Can you work these out from the model? Positions are in its coordinate system, mm. A direction names the side the tool comes from. Coordinates: 2 decimals unless noted, no trailing zeros. Write each loop counter-clockwise with the first axis right and the second up, starting at its lowest first coordinate (ties: lowest second). Pieces come first, ordered by that corner, then holes. Notation, with made-up numbers: (9.25, 34) - (56.25, 34) arc R29 cw to (56.25, 71) - close; hole circle Ø7 at (42.5, -37.5). An arc over 180 degrees is marked (long way). Write each question's results on one line, items separated by ' | '. Start each with the question number.
```python
from build123d import *


with BuildPart() as f1:
    # F0 (on Top) → F1 (revolve)
    with BuildSketch(Plane.XY):
        with BuildLine():
            Line((-8.1, 12.624975), (0, 0))
            Line((0, 0), (3.5, 0))
            Line((3.5, 0), (3.5, 7))
            Line((3.5, 7), (-1.81, 7))
            Line((-1.81, 7), (-1.81, 10.05))
            Line((-1.81, 10.05), (0.49, 10.05))
            Line((0.49, 10.05), (-1.356164, 21.907136))
            Line((-1.356164, 21.907136), (-12.356164, 21.907136))
            Line((-12.356164, 21.907136), (-12.356164, 21.31))
            ThreePointArc((-12.356164, 21.31), (-7.520242, 18.294486), (-8.1, 12.624975))
        make_face()
    revolve(axis=Axis((-12.356164, 10.953568, 0), (0, -1, 0)))


solid = f1.part
```
Q1. Thinking about a two-plate mould opening in Z: for faces 3 (the face through (-18.014, 10.432, 0.249)), 4 (the face through (-9.1, 7, -10.3)), 5 (the face through (-21.645, 17.379, -7.122)), which applies, pulls with the +Z half, pulls with the -Z half, needs draft (parallel to the pull), parting line crosses it, or undercut?
Q2. If we section it at A-A (y = 1.5): Please give me the cut outline in (x, z), then the cut area to 3 significant figures.
Q3. If we section it at C-C (y = 11.25): Please give me the cut outline in (x, z), then the cut area to 3 significant figures.
Q4. If we section it at B-B (x = 1.5): Please give me the cut outline in (y, z), then the cut area to 3 significant figures.
Q5. I'm going to push flat-ended pins straight in: pin 1 Ø1.5 at (x, y) = (-15, 17) entering from +Z; pin 2 Ø8 at (x, z) = (-11, 6) entering from -Y; pin 3 Ø5 at (x, z) = (-6, -4) entering from -Y. Where does each tip first touch, or does it pass through?
Q6. For faces 1 (the face through (-22.892, 8.546, 0.464)), 2 (the face through (2.77, 3.55, 4.76)), which set-ups out of +Z, -Z, +X, -X, +Y, -Y let a thin tool reach every point of the face, with its end or its side?
Q7. I need wall thicknesses on line 1 along X through (y, z) = (1.75, 9.5); line 2 along X through (y, z) = (7.75, 2); line 3 along Y through (x, z) = (-26, -4). Which ranges of each line are inside material? Lowest first, please. Write a range as from..to.
Answer list:
1) face 3: undercut | face 4: needs draft | face 5: parting line crosses it
2) outline: circle Ø31.71 at (-12.36, 0); hole circle Ø22.79 at (-12.36, 0) | area: 382 mm2
3) outline: circle Ø25.32 at (-12.36, 0); hole circle Ø10.28 at (-12.36, 0) | area: 421 mm2
4) outline: (0, -7.71) - (7, -7.71) - (7, 7.71) - (0, 7.71) - close | area: 108 mm2
5) pin 1: stops at z = 11.66 | pin 2: stops at y = 3.44 | pin 3: stops at y = 3.66
6) face 1: none | face 2: +Y, -Y
7) line 1: x = -25.05..-18.35, -6.36..0.34 | line 2: x = -22.71..-19.46, -5.25..-2 | line 3: y = 0..7
